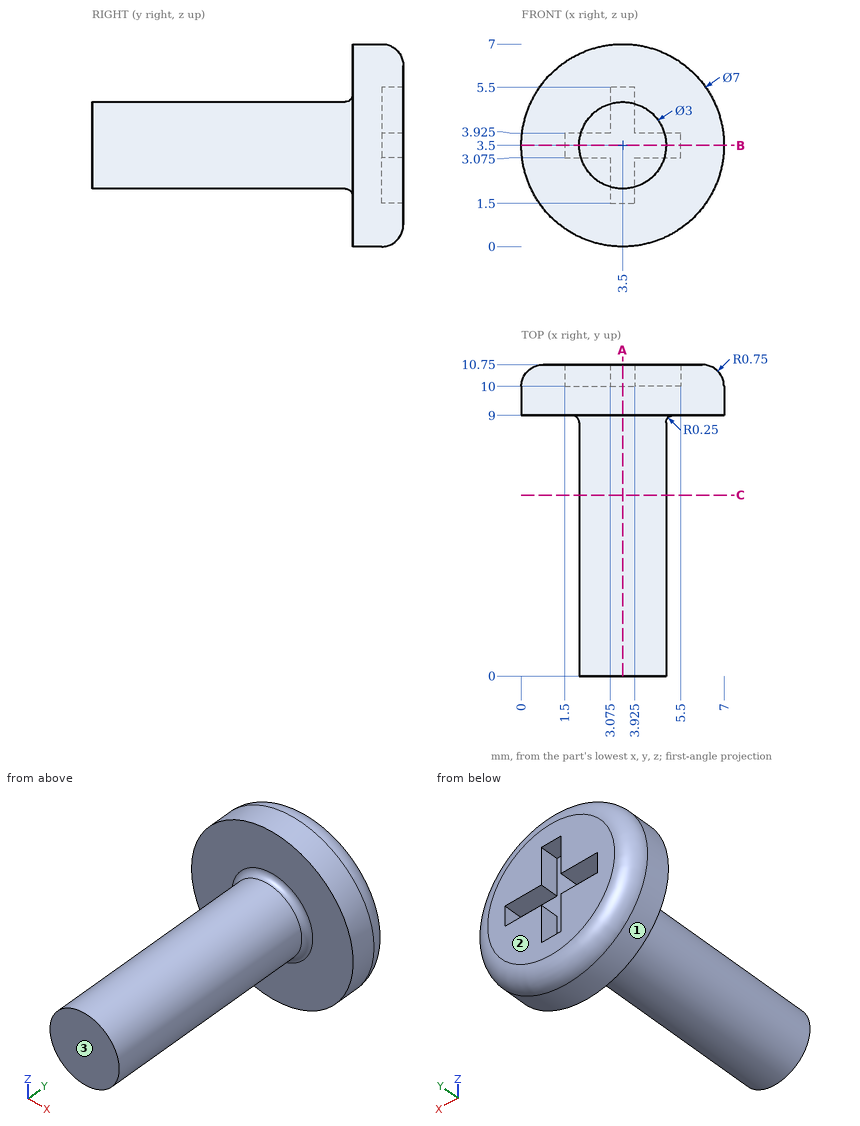
Study the drawing (mm; zero at the part's minimum x, y, z) and answer. Round coordinates to 2 decimals unless told otherwise and drop trailing zeros. Write each loop counter-clockwise with the first axis right and the second up, starting at its lowest first coordinate (ties: lowest second). Pieces come first, ordered by that corner, then holes.
1) A cutting plane is placed at A-A on x = 3.5. Determine the outline of the cut face in (y, z).
2) A cutting plane is placed at C-C on y = 6.25. Determine the outline of the cut face in (x, z), and give its area (3 significant figures).
3) Flat-ended cylindrical pins translate along their axes: P1, Ø0.6, axis at x = 2.5, y = 10.5, coming from the -Z side; P2, Ø2, axis at x = 4.5, z = 4.5, coming from the -Y side; P3, Ø0.6, axis at y = 10.5, z = 3.5, coming from the +X side; P4, Ø0.8, axis at x = 3.5, y = 10.5, coming from the +Z side. Find the tip coordinate at first contact, or state that the pin passes through.
4) Determine the mould class of the marked faces 1, 2 and 3 for opening direction Y: pulls with the +Y half, pulls with the -Y half, needs draft (parallel to the pull), parting line crosses it, or undercut.
5) Consider probe 1 along Y at (x, z) = (3, 1); probe 2 along Y at (x, z) = (4, 3.75); probe 3 along X at (y, z) = (5, 3.25). Determine where each line is inside the solid, lowest interval first.
6) A cutting plane is placed at B-B on z = 3.5. Determine the outline of the cut face in (x, y).
Entries:
1. outline: (0, 2) - (8.75, 2) arc R0.25 cw to (9, 1.75) - (9, 0) - (10, 0) arc R0.75 ccw to (10.75, 0.75) - (10.75, 1.5) - (10, 1.5) - (10, 5.5) - (10.75, 5.5) - (10.75, 6.25) arc R0.75 ccw to (10, 7) - (9, 7) - (9, 5.25) arc R0.25 cw to (8.75, 5) - (0, 5) - close
2. outline: circle Ø3 at (3.5, 3.5)
2. area: 7.07 mm2
3. P1: stops at z = 0.15
3. P2: stops at y = 0
3. P3: stops at x = 6.97
3. P4: stops at z = 6.99
4. face 1: needs draft
4. face 2: pulls with the +Y half
4. face 3: pulls with the -Y half
5. probe 1: y = 9 to 10.75
5. probe 2: y = 0 to 10
5. probe 3: x = 2.02 to 4.98
6. outline: (0, 9) - (1.75, 9) arc R0.25 cw to (2, 8.75) - (2, 0) - (5, 0) - (5, 8.75) arc R0.25 cw to (5.25, 9) - (7, 9) - (7, 10) arc R0.75 ccw to (6.25, 10.75) - (5.5, 10.75) - (5.5, 10) - (1.5, 10) - (1.5, 10.75) - (0.75, 10.75) arc R0.75 ccw to (0, 10) - close
